```python
from build123d import *

# Parameters (mm, degrees)
F1_DEPTH = 7.9
F2_R     = 3.95
F3_DEPTH = 10.9
F4_R     = 1
F5_R     = 1


with BuildPart() as f1:
    # F0 (on Top) → F1 (new body)
    with BuildSketch(Plane.XY):
        with BuildLine():
            Line((9.5, -8.1240384046), (9.5, 8.1240384046))
            ThreePointArc((9.5, 8.1240384046), (6.6733417963, 10.5696030801), (3.25, 12.0701077046))
            ThreePointArc((3.25, 12.0701077046), (1.85, 0), (3.25, -12.0701077046))
            ThreePointArc((3.25, -12.0701077046), (6.6733417963, -10.5696030801), (9.5, -8.1240384046))
        make_face()
    extrude(amount=F1_DEPTH)



with BuildPart() as f1b:
    # F0 (on Top) → F1, piece 2 (new body)
    with BuildSketch(Plane.XY):
        with BuildLine():
            ThreePointArc((-3.25, 12.0701077046), (-6.6733417963, 10.5696030801), (-9.5, 8.1240384046))
            Line((-9.5, 8.1240384046), (-9.5, -8.1240384046))
            ThreePointArc((-9.5, -8.1240384046), (-6.6733417963, -10.5696030801), (-3.25, -12.0701077046))
            ThreePointArc((-3.25, -12.0701077046), (-1.85, 0), (-3.25, 12.0701077046))
        make_face()
    extrude(amount=F1_DEPTH)


with BuildPart() as f1_1:
    add(f1.part)

    add(f1b.part)  # F3 merges F1b
    # F2 (on face) → F3 (join)
    with BuildSketch(Plane(origin=(0, 0, 0), x_dir=(1, 0, 0), z_dir=(0, 0, -1))):
        with BuildLine():
            Line((-9.5, 8.1240384046), (-9.5, -8.1240384046))
            ThreePointArc((-9.5, -8.1240384046), (0, -12.5), (9.5, -8.1240384046))
            Line((9.5, -8.1240384046), (9.5, 8.1240384046))
            ThreePointArc((9.5, 8.1240384046), (0, 12.5), (-9.5, 8.1240384046))
        make_face()
        Circle(F2_R, mode=Mode.SUBTRACT)
    extrude(amount=F3_DEPTH)

    # F4
    f4_edges = [f1_1.edges().sort_by_distance(p)[0] for p in [
        (-9.5, -8.124038, -1.5),
        (9.5, -8.124038, -1.5),
        (9.5, 8.124038, -1.5),
        (-9.5, 8.124038, -1.5),
    ]]
    fillet(f4_edges, radius=F4_R)

    # F5
    f5_edges = [f1_1.edges().sort_by_distance(p)[0] for p in [
        (-9.5, 0, 7.9),
        (6.505865, -10.673506, 7.9),
    ]]
    fillet(f5_edges, radius=F5_R)


solid = f1_1.part
```
Build history of the part. All positions in model axes, mm. A direction names the side the tool comes from. Coordinates: 2 decimals unless noted, no trailing zeros. Write each loop counter-clockwise with the first axis right and the second up, starting at its lowest first coordinate (ties: lowest second). Pieces come first, ordered by that corner, then holes.
1. Drop flat-ended pins along their axis: pin 1 (3 mm diameter, centred on x = 0, y = -1.5, fed in from +Z); pin 2 (1.7 mm diameter, centred on x = 3, y = 0, fed in from -Z); pin 3 (8 mm diameter, centred on x = -5.5, z = -7.5, fed in from -Y); pin 4 (6 mm diameter, centred on x = -1, z = 4, fed in from +Y). Give the stop position or say it passes through.
Answer block:
pin 1: passes through
pin 2: stops at z = 0
pin 3: stops at y = -12.41
pin 4: stops at y = 12.07
2. Band-saw the part on B-B, the plane z = 2.75. Give the cut face in (x, y).
Answer block:
outline: (-9.5, -7.75) arc R1 ccw to (-9.24, -8.42) arc R12.5 ccw to (-3.25, -12.07) arc R52.73 ccw to (-3.25, 12.07) arc R12.5 ccw to (-9.24, 8.42) arc R1 ccw to (-9.5, 7.75) - close; (3.25, -12.07) arc R12.5 ccw to (9.24, -8.42) arc R1 ccw to (9.5, -7.75) - (9.5, 7.75) arc R1 ccw to (9.24, 8.42) arc R12.5 ccw to (3.25, 12.07) arc R52.73 ccw to start
3. Drill centre lines: probe 1 along X at (y, z) = (0, -5.25); probe 2 along Z at (x, y) = (-0.5, -5.75); probe 3 along Y at (x, z) = (2.75, -2.5). Where is each one in solid material? Low to high.
Answer block:
probe 1: x = -9.5 to -3.95, 3.95 to 9.5
probe 2: z = -10.9 to 0
probe 3: y = -12.19 to -2.84, 2.84 to 12.19
4. 3-axis set-ups, long thin cutter, end or side, ignore diameter. For faces 1 (the flat face through (9.5, 0, -2)), 2 (the flat face through (0, -8, 0)), 3 (the cylindrical face through (1.85, 0.17, 3.89)), 4 (the flat face through (3, 0, 0)), 5 (the flat face through (0, 9, 0)): which of +Z, -Z, +X, -X, +Y, -Y reach the whole face in a straight line?
Answer block:
face 1: +Z, -Z, +X, +Y, -Y
face 2: +Z, -Y
face 3: +Z
face 4: -Z
face 5: +Z, +Y
5. Band-saw the part on C-C, the plane x = 0. Give the cut face in (y, z).
Answer block:
outline: (-12.5, -10.9) - (-3.95, -10.9) - (-3.95, 0) - (-12.5, 0) - close; (3.95, -10.9) - (12.5, -10.9) - (12.5, 0) - (3.95, 0) - close
6. Band-saw the part on D-D, the plane z = -0.75. Give the cut face in (x, y), and give its area (3 significant figures).
Answer block:
outline: (-9.5, -7.75) arc R1 ccw to (-9.24, -8.42) arc R12.5 ccw to (9.24, -8.42) arc R1 ccw to (9.5, -7.75) - (9.5, 7.75) arc R1 ccw to (9.24, 8.42) arc R12.5 ccw to (-9.24, 8.42) arc R1 ccw to (-9.5, 7.75) - close; hole circle Ø7.9 at (0, 0)
area: 375 mm2
7. Band-saw the part on A-A, the plane y = 0. Give the cut face in (x, z), and give its area (3 significant figures).
Answer block:
outline: (-9.5, -10.9) - (-3.95, -10.9) - (-3.95, 0) - (-1.85, 0) - (-1.85, 7.9) - (-8.5, 7.9) arc R1 ccw to (-9.5, 6.9) - close; (1.85, 0) - (3.95, 0) - (3.95, -10.9) - (9.5, -10.9) - (9.5, 6.9) arc R1 ccw to (8.5, 7.9) - (1.85, 7.9) - close
area: 241 mm2
